Source: CAD feature listing. Evaluate the final solid. Frame: model axes, mm. Face numbers are marked on the shaded views. A direction names the side the tool comes from. Round coordinates to 2 decimals unless told otherwise and drop trailing zeros. Write each loop counter-clockwise with the first axis right and the second up, starting at its lowest first coordinate (ties: lowest second). Pieces come first, ordered by that corner, then holes. Notation, with made-up numbers: M -37,0.5 L 15,0.5 A17 cw 15,29.5 Z; hole C 27,-40 d10. An arc over 180 degrees is marked long. Use a Markdown table: item, result.
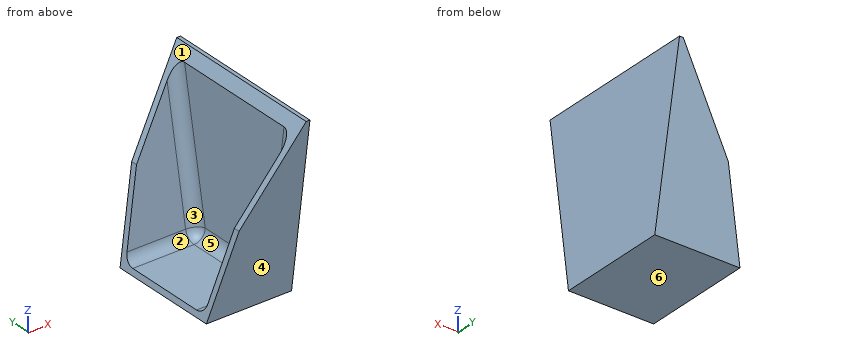
```python
from build123d import *

# Parameters (mm, degrees)
F1_DEPTH      = 100
F3_DEPTH      = 90
F4_R          = 10
F6_DEPTH      = 65.794616
F6_DEPTH_BACK = 84.207384


with BuildPart() as f1:
    # F0 (on Right) → F1 (new body)
    with BuildSketch(Plane.YZ):
        Polygon((84.206384, 102.410072), (-65.793616, 102.410072), (-44.478415, -47.589928), (55.521585, -47.589928), align=None)
    extrude(amount=F1_DEPTH)

    # F2 (on face) → F3 (cut)
    with BuildSketch(Plane(origin=(0, 0, 0), x_dir=(0, -1, 0), z_dir=(-1, 0, 0))):
        Polygon((60.0917, 102.410072), (-78.619334, 102.410072), (-50.892521, -42.580376), (39.917622, -42.711261), align=None)
    extrude(amount=-F3_DEPTH, mode=Mode.SUBTRACT)

    # F4
    f4_edges = [f1.edges().sort_by_distance(p)[0] for p in [
        (45, 50.892521, -42.580376),
        (90, 5.48745, -42.645818),
        (45, -39.917622, -42.711261),
        (90, 64.755927, 29.914848),
        (90, -50.004661, 29.849406),
    ]]
    fillet(f4_edges, radius=F4_R)

    # F5 (on Front) → F6 (cut, two sides)
    with BuildSketch(Plane.XZ) as f6_sk:
        Polygon((-27.018974, -66.479579), (18.04512, -66.479579), (44.833042, 25.719849), (101.288192, 109.236158), (-27.018974, 105.970137), align=None)
    extrude(amount=F6_DEPTH, mode=Mode.SUBTRACT)
    extrude(f6_sk.sketch, amount=-F6_DEPTH_BACK, mode=Mode.SUBTRACT)


solid = f1.part
```
Q1. Line query: L1, parallel to X at y = -17.5, z = 2.5; L2, parallel to Z at x = 63, y = -12; L3, parallel to Y at x = 79.5, z = -25.5. Output: solid intervals per line, ascending.
Results are:
| item | result |
|---|---|
| L1 | 90 to 100 |
| L2 | -47.59 to -42.67 |
| L3 | -47.62 to -42.31, 54.16 to 59.75 |
Q2. First-contact query: pin 1 Ø12 at (x, z) = (60, -23.5) entering from -Y; pin 2 Ø5 at (x, z) = (56, 11) entering from +Y; pin 3 Ø5 at (x, z) = (57, 43) entering from +Y. Flat tips, straight axial feed; report the tip coordinate or a pass-through.
Results are:
| item | result |
|---|---|
| pin 1 | y = -48.75 |
| pin 2 | y = 67.2 |
| pin 3 | y = 73.28 |
Q3. Mould query, pull axis Y, two halves, no side actions, for the marked faces 1, 2, 3 and 4. Classes: +Y half, -Y half, draft (parallel to the pull), parting line (faces both ways), or undercut.
Results are:
| item | result |
|---|---|
| face 1 | draft |
| face 2 | undercut |
| face 3 | undercut |
| face 4 | -Y half |
Q4. Section C-C on x = 94. Return loops of the section in (y, z).
Results are:
| item | result |
|---|---|
| outline | M -65.23,98.45 L -44.48,-47.59 L 55.52,-47.59 L 83.45,98.45 Z |
Q5. Section A-A on x = 75.5. Return loops of the section in (y, z).
Results are:
| item | result |
|---|---|
| outline | M -61.34,71.09 L -44.48,-47.59 L 55.52,-47.59 L 78.22,71.09 L 72.63,71.09 L 52.44,-34.47 A10 cw 42.64,-42.59 L -31.2,-42.7 A10 cw -41.12,-34.08 L -55.74,71.09 Z |
Q6. Reachability of the marked faces 5 and 6 from +Z, -Z, +X, -X, +Y, -Y: full face, straight path, thin tool, end or side. Return the list, or none.
Results are:
| item | result |
|---|---|
| face 5 | +Z, -X |
| face 6 | -Z, +X, -X, +Y, -Y |
Q7. Section B-B on x = 84.5. Return loops of the section in (y, z).
Results are:
| item | result |
|---|---|
| outline | M -63.23,84.4 L -44.48,-47.59 L 55.52,-47.59 L 80.76,84.4 L 74.09,84.4 L 51.39,-34.27 A8.93 cw 42.63,-41.52 L -31.2,-41.63 A8.93 cw -40.06,-33.93 L -56.51,84.4 Z |
